Part model, mm, in its own coordinate system. A direction names the side the tool comes from. Coordinates: 2 decimals unless noted, no trailing zeros. Write each loop counter-clockwise with the first axis right and the second up, starting at its lowest first coordinate (ties: lowest second). Pieces come first, ordered by that corner, then holes. Notation, with made-up numbers: M 49.25,75 L 84.25,75 A22 cw 84.25,96 Z; hole C -39.5,19 d8. An arc over 180 degrees is marked long. Use a Markdown table: item, result. Add a question column.
Q1. Mould opens along Y. For faces 1 (the cylindrical face through (-40.4, 12.4, 3.2)), 2 (the flat face through (-64.05, 52.6, 3.13)), 3 (the flat face through (-46.841, 0, 3)) say: released by +Y, released by -Y, zero draft, split by the parting line, or undercut.
Q2. Slice it at D-D on y = 43. Write the cut outline in (x, z), then the cut area to 3 significant figures.
Q3. Pin check, flat tips, straight feed: pin 1 Ø1.9 at (y, z) = (4.5, 2) entering from -X; pin 2 Ø1.5 at (x, z) = (34.5, 2) entering from +Y; pin 3 Ø1 at (x, y) = (-31, 42.5) entering from -Z; pin 4 Ø3 at (y, z) = (-3.5, 3.5) entering from -X. Stop position of each tip, or through.
Q4. Tool access for faces 4 (the flat face through (41.42, -2, 3)), 5 (the cylindrical face through (-48.95, -12.32, 3.22)), 6 (the flat face through (-49.34, 73.31, 3.13)), 7 (the flat face through (-50.123, 83.41, 3.131)), 8 (the cylindrical face through (-54.053, -17.092, 3.131)): list every direction of +Z, -Z, +X, -X, +Y, -Y with a clear straight run to the whole face (end or side of a thin tool).
Q5. Slice it at B-B on z = 2. Count the separate pieces of the cut face and the enclosed holes in it, then the cut area to 3 significant figures.
Q6. Wall check: L1, parallel to X at y = 9, z = 5.5; L2, parallel to X at y = -7.5, z = 0.5; L3, parallel to X at y = 52.5, z = 4. Give the ranges that are in metal, low to high. Write a range as from..to.
Q7. Slice it at C-C on x = 49. Write the cut outline in (y, z), then the cut area to 3 significant figures.
Q8. Slice it at A-A on x = -49. Write the cut outline in (y, z).
from build123d import *

# Parameters (mm, degrees)
EXTRUDE1_DEPTH     = 6.35
CUT_EXTRUDE3_REACH = 8.35
FILLET1_R          = 9.525


with BuildPart() as part:
    # Sketch1 → Extrude1 (new body)
    with BuildSketch(Plane.XY):
        with BuildLine():
            Line((-41.42, 12.7), (-41.42, -12.7))
            ThreePointArc((-41.42, -12.7), (-42.907897552, -16.292102448), (-46.5, -17.78))
            Line((-46.5, -17.78), (-51.5, -17.78))
            ThreePointArc((-51.5, -17.78), (-54.085377818, -17.072896242), (-55.951019269, -15.148433677))
            Line((-55.951019269, -15.148433677), (-83.74924785, 35.386098748))
            Line((-83.74924785, 35.386098748), (-69.180406366, 56.192560673))
            Line((-69.180406366, 56.192560673), (-58.777175404, 48.908139931))
            ThreePointArc((-58.777175404, 48.908139931), (-41.0895237, 52.026950152), (-44.208333921, 69.714601856))
            Line((-44.208333921, 69.714601856), (-54.611564883, 76.999022598))
            Line((-54.611564883, 76.999022598), (-40.0427234, 97.805484523))
            Line((-40.0427234, 97.805484523), (56.58, 30.149525236))
            Line((56.58, 30.149525236), (56.58, -12.7))
            ThreePointArc((56.58, -12.7), (55.092102448, -16.292102448), (51.5, -17.78))
            Line((51.5, -17.78), (46.5, -17.78))
            ThreePointArc((46.5, -17.78), (42.907897552, -16.292102448), (41.42, -12.7))
            Line((41.42, -12.7), (41.42, 12.7))
            ThreePointArc((41.42, 12.7), (0, 28.068579909), (-41.42, 12.7))
        make_face()
    extrude(amount=EXTRUDE1_DEPTH)

    # Sketch4 → Cut-Extrude3 (cut, up to next)
    with BuildSketch(Plane.XY.offset(6.35), mode=Mode.PRIVATE) as cut_extrude3_sk1:
        with BuildLine():
            Line((-51.159, -10.16), (-51.159, 10.16))
            ThreePointArc((-51.159, 10.16), (-49, 12.319), (-46.841, 10.16))
            Line((-46.841, 10.16), (-46.841, -10.16))
            ThreePointArc((-46.841, -10.16), (-49, -12.319), (-51.159, -10.16))
        make_face()
    cut_extrude3_tool1 = extrude(cut_extrude3_sk1.sketch, amount=-CUT_EXTRUDE3_REACH, mode=Mode.PRIVATE) & part.part
    add(cut_extrude3_tool1.solids().sort_by_distance((-49, 0, 6.35))[0], mode=Mode.SUBTRACT)
    # Sketch4 → Cut-Extrude3 (cut, up to next)
    with BuildSketch(Plane.XY.offset(6.35), mode=Mode.PRIVATE) as cut_extrude3_sk2:
        with BuildLine():
            Line((2.159, 38.84), (2.159, 59.16))
            ThreePointArc((2.159, 59.16), (0, 61.319), (-2.159, 59.16))
            Line((-2.159, 59.16), (-2.159, 38.84))
            ThreePointArc((-2.159, 38.84), (0, 36.681), (2.159, 38.84))
        make_face()
    cut_extrude3_tool2 = extrude(cut_extrude3_sk2.sketch, amount=-CUT_EXTRUDE3_REACH, mode=Mode.PRIVATE) & part.part
    add(cut_extrude3_tool2.solids().sort_by_distance((0, 49, 6.35))[0], mode=Mode.SUBTRACT)
    # Sketch4 → Cut-Extrude3 (cut, up to next)
    with BuildSketch(Plane.XY.offset(6.35), mode=Mode.PRIVATE) as cut_extrude3_sk3:
        with BuildLine():
            Line((51.159, -10.16), (51.159, 10.16))
            ThreePointArc((51.159, 10.16), (49, 12.319), (46.841, 10.16))
            Line((46.841, 10.16), (46.841, -10.16))
            ThreePointArc((46.841, -10.16), (49, -12.319), (51.159, -10.16))
        make_face()
    cut_extrude3_tool3 = extrude(cut_extrude3_sk3.sketch, amount=-CUT_EXTRUDE3_REACH, mode=Mode.PRIVATE) & part.part
    add(cut_extrude3_tool3.solids().sort_by_distance((49, 0, 6.35))[0], mode=Mode.SUBTRACT)

    # Fillet1
    fillet1_edges = [part.edges().sort_by_distance(p)[0] for p in [
        (-41.42, 12.7, 3.175),
        (-83.74924785, 35.386098748, 3.175),
        (-40.0427234, 97.805484523, 3.175),
        (56.58, 30.149525236, 3.175),
        (41.42, 12.7, 3.175),
    ]]
    fillet(fillet1_edges, radius=FILLET1_R)


solid = part.part
Recorded:
| question | item | result |
|---|---|---|
| 1 | face 1 | released by -Y |
| 1 | face 2 | released by +Y |
| 1 | face 3 | undercut |
| 2 | outline | M -78.42,0 L -2.16,0 L -2.16,6.35 L -78.42,6.35 Z; M 2.16,0 L 38.23,0 L 38.23,6.35 L 2.16,6.35 Z |
| 2 | area | 713 mm² |
| 3 | pin 1 | x = -67.28 |
| 3 | pin 2 | y = 46.14 |
| 3 | pin 3 | z = 0 |
| 3 | pin 4 | x = -63.18 |
| 4 | face 4 | +Z, -Z, -Y |
| 4 | face 5 | +Z, -Z |
| 4 | face 6 | +Z, -Z, -X |
| 4 | face 7 | +Z, -Z, -X, +Y |
| 4 | face 8 | +Z, -Z, -X, -Y |
| 5 | separate pieces | 1 |
| 5 | enclosed holes | 3 |
| 5 | area | 6,490 mm² |
| 6 | L1 | -69.23..-51.16, -46.84..-41.38, 41.38..46.84, 51.16..56.58 |
| 6 | L2 | -60.16..-51.16, -46.84..-41.42, 41.42..46.84, 51.16..56.58 |
| 6 | L3 | -71.77..-63.91, -40.77..-2.16, 2.16..24.66 |
| 7 | outline | M -17.78,0 L -12.32,0 L -12.32,6.35 L -17.78,6.35 Z; M 12.32,0 L 35.46,0 L 35.46,6.35 L 12.32,6.35 Z |
| 7 | area | 182 mm² |
| 8 | outline | M -17.78,0 L -12.32,0 L -12.32,6.35 L -17.78,6.35 Z; M 12.32,0 L 46.86,0 L 46.86,6.35 L 12.32,6.35 Z; M 73.07,0 L 85.01,0 L 85.01,6.35 L 73.07,6.35 Z |
